Read the model definition and answer for the solid it produces. Units are mm, in the model's axes. Face numbers are marked on the shaded views. Coordinates: 2 decimals unless noted, no trailing zeros. Order: outer loops, then holes, each group sorted by start corner. A loop starts at its lowest first (then second) coordinate and runs counter-clockwise, first axis right, second up. Notation, with made-up numbers: (28, -25.5) -> (54, -25.5) arc R15 cw to (54, 0.5) -> close; hole circle Ø8 at (-36.5, -2.75). An arc over 180 degrees is marked (long way). Answer in a Markdown table with one row per item.
from build123d import *

# Parameters (mm, degrees)
BASE_FLANGE1_DEPTH      = 80
CUT_EXTRUDE1_DEPTH      = 219.886820069
CUT_EXTRUDE1_DEPTH_BACK = 219.886820069
SKETCH7_R               = 1.5
CUT_EXTRUDE3_DEPTH      = 0.7
SKETCH8_R               = 1.5
CUT_EXTRUDE4_DEPTH      = 0.7
SKETCH9_R               = 1.5
CUT_EXTRUDE5_DEPTH      = 0.7


# Sheet-metal steps are written as plain solids
with BuildPart() as part:
    # Sketch1 → Base-Flange1 (new body)
    with BuildSketch(Plane(origin=(0, 0, 0), x_dir=(1, 0, 0), z_dir=(0, 1, 0))):
        with BuildLine():
            Line((169, 56.9), (1.4, 56.9))
            ThreePointArc((1.4, 56.9), (0.410050506, 56.489949494), (0, 55.5))
            Line((0, 55.5), (0, 0))
            Line((0, 0), (0, -55.5))
            ThreePointArc((0, -55.5), (0.410050506, -56.489949494), (1.4, -56.9))
            Line((1.4, -56.9), (169, -56.9))
            Line((169, -56.9), (169, -56.2))
            Line((169, -56.2), (1.4, -56.2))
            ThreePointArc((1.4, -56.2), (0.905025253, -55.994974747), (0.7, -55.5))
            Line((0.7, -55.5), (0.7, 0))
            Line((0.7, 0), (0.7, 55.5))
            ThreePointArc((0.7, 55.5), (0.905025253, 55.994974747), (1.4, 56.2))
            Line((1.4, 56.2), (169, 56.2))
            Line((169, 56.2), (169, 56.9))
        make_face()
    extrude(amount=BASE_FLANGE1_DEPTH)

    # Sketch6 → Cut-Extrude1 (cut, two sides: drawn at the far end of the back side and taken through both)
    with BuildSketch(Plane.XY.offset(56.9).offset(-CUT_EXTRUDE1_DEPTH_BACK)):
        Polygon((169, 50), (169, 0), (119, 0), align=None)
    extrude(amount=CUT_EXTRUDE1_DEPTH + CUT_EXTRUDE1_DEPTH_BACK, mode=Mode.SUBTRACT)

    # Sketch7 → Cut-Extrude3 (cut)
    with BuildSketch(Plane.XY.offset(56.9)):
        with Locations((159, 70)):
            Circle(SKETCH7_R)
        with Locations((119, 70)):
            Circle(SKETCH7_R)
    extrude(amount=-CUT_EXTRUDE3_DEPTH, mode=Mode.SUBTRACT)

    # Sketch8 → Cut-Extrude4 (cut)
    with BuildSketch(Plane.XY.offset(-56.9)):
        with Locations((139, 70)):
            Circle(SKETCH8_R)
    extrude(amount=CUT_EXTRUDE4_DEPTH, mode=Mode.SUBTRACT)

    # Sketch9 → Cut-Extrude5 (cut)
    with BuildSketch(Plane.ZY):
        with Locations((-51, 29)):
            Circle(SKETCH9_R)
        with Locations((-14, 29)):
            Circle(SKETCH9_R)
        with Locations(Location((14, 29, 0), (0, 0, 180))):
            Circle(SKETCH9_R)
        with Locations(Location((51, 29, 0), (0, 0, 180))):
            Circle(SKETCH9_R)
    extrude(amount=-CUT_EXTRUDE5_DEPTH, mode=Mode.SUBTRACT)


solid = part.part
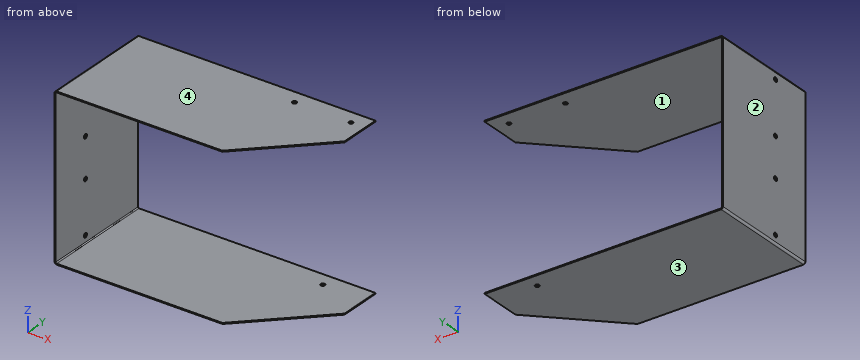
Q1. The part is cut by section C-C (z = -41.5). Write down the section's boundary in (x, y), then the cut area to 3 significant figures.
Outcome:
| item | result |
|---|---|
| outline | (0, 0) -> (0.7, 0) -> (0.7, 80) -> (0, 80) -> close |
| area | 56.0 mm² |
Q2. The part is cut by section A-A (x = 97). Write down the section's boundary in (y, z).
Outcome:
| item | result |
|---|---|
| outline | (0, -56.9) -> (80, -56.9) -> (80, -56.2) -> (0, -56.2) -> close; (0, 56.2) -> (80, 56.2) -> (80, 56.9) -> (0, 56.9) -> close |
Q3. Consider line 1 (Z direction, x = 103, y = 55.5); line 2 (Y direction, x = 0.55, z = 51); line 3 (X direction, y = 70, z = 56.45). Determine where each line is inside the solid, lowest interval first.
Outcome:
| item | result |
|---|---|
| line 1 | -56.9 to -56.2, 56.2 to 56.9 |
| line 2 | 0 to 27.5, 30.5 to 80 |
| line 3 | 0.37 to 117.5, 120.5 to 157.5, 160.5 to 169 |
Q4. The part is cut by section B-B (y = 64). Write down the section's boundary in (x, z), then the cut area to 3 significant figures.
Outcome:
| item | result |
|---|---|
| outline | (0, -55.5) arc R1.4 ccw to (1.4, -56.9) -> (169, -56.9) -> (169, -56.2) -> (1.4, -56.2) arc R0.7 cw to (0.7, -55.5) -> (0.7, 55.5) arc R0.7 cw to (1.4, 56.2) -> (169, 56.2) -> (169, 56.9) -> (1.4, 56.9) arc R1.4 ccw to (0, 55.5) -> close |
| area | 315 mm² |
Q5. For a pull along Z with two mould halves and no side action, classify the marked faces 1, 2, 3 and 4 as pulls with the +Z half, pulls with the -Z half, needs draft (parallel to the pull), parting line crosses it, or undercut.
Outcome:
| item | result |
|---|---|
| face 1 | undercut |
| face 2 | needs draft |
| face 3 | pulls with the -Z half |
| face 4 | pulls with the +Z half |
Q6. Given pin 1 (2.5 mm diameter, centred on y = 29, z = -14, fed in from -X); pin 2 (4 mm diameter, centred on y = 12.5, z = 18, fed in from +X), each flat-ended and moving along its own axis, determine where each tip first touches the part or whether it passes through.
Outcome:
| item | result |
|---|---|
| pin 1 | through |
| pin 2 | x = 0.7 |
